```python
from build123d import *

# Parameters (mm, degrees)
SKETCH_1_W               = 8
SKETCH_1_H               = 10
SKETCH_1_R               = 1.5
EXTRUDE_1_DEPTH          = 0.5
SM_START                 = -5
SM_EDGE_FLANGE_1_DEPTH   = 10
SM_EDGE_FLANGE_1_2_DEPTH = 10
SM_EDGE_FLANGE_2_DEPTH   = 10
SM_EDGE_FLANGE_2_2_DEPTH = 10
FILLET_1_R               = 2
SKETCH_18_R              = 1.5
CUT_EXTRUDE_1_DEPTH      = 10


# Read off the part's stored shape, not the designer's step: Ребро-кромка1, Ребро-кромка2
with BuildPart() as part:
    # Sketch 1 → Бобышка-Вытянуть1 (new body)
    with BuildSketch(Plane(origin=(0, 0, 0), x_dir=(1, 0, 0), z_dir=(0, 1, 0))):
        Rectangle(SKETCH_1_W, SKETCH_1_H)
        with Locations(Location((0, 0, 0), (0, 0, 270))):
            Circle(SKETCH_1_R, mode=Mode.SUBTRACT)
    extrude(amount=EXTRUDE_1_DEPTH)

    # Ребро-кромка1 outline → Ребро-кромка1 (cut)
    with BuildSketch(Plane.XY.offset(SM_START)):
        with BuildLine():
            ThreePointArc((-2.75383711, 0), (-3.25383711, 0.133974596), (-3.619862514, 0.5))
            Line((-3.619862514, 0.5), (-4, 0.5))
            Line((-4, 0.5), (-4, 0))
            Line((-4, 0), (-2.75383711, 0))
        make_face()
        with BuildLine():
            ThreePointArc((3.619862514, 0.5), (3.25383711, 0.133974596), (2.75383711, 0))
            Line((2.75383711, 0), (4, 0))
            Line((4, 0), (4, 0.5))
            Line((4, 0.5), (3.619862514, 0.5))
        make_face()
    extrude(amount=SM_EDGE_FLANGE_1_DEPTH, mode=Mode.SUBTRACT)

    # Sm Edge Flange 1 2 outline → Sm Edge Flange 1 2 (add)
    with BuildSketch(Plane.XY.offset(SM_START)):
        with BuildLine():
            Line((-2.129864257, 5.638155725), (-3.693529731, 1.342020143))
            ThreePointArc((-3.693529731, 1.342020143), (-3.750031808, 0.912844257), (-3.619862514, 0.5))
            Line((-3.619862514, 0.5), (-2.75383711, 0.5))
            ThreePointArc((-2.75383711, 0.5), (-3.163413133, 0.713211782), (-3.223683421, 1.171010072))
            Line((-3.223683421, 1.171010072), (-1.660017947, 5.467145653))
            Line((-1.660017947, 5.467145653), (-2.129864257, 5.638155725))
        make_face()
        with BuildLine():
            ThreePointArc((3.223683421, 1.171010072), (3.163413133, 0.713211782), (2.75383711, 0.5))
            Line((2.75383711, 0.5), (3.619862514, 0.5))
            ThreePointArc((3.619862514, 0.5), (3.750031808, 0.912844257), (3.693529731, 1.342020143))
            Line((3.693529731, 1.342020143), (2.129864257, 5.638155725))
            Line((2.129864257, 5.638155725), (1.660017947, 5.467145653))
            Line((1.660017947, 5.467145653), (3.223683421, 1.171010072))
        make_face()
    extrude(amount=SM_EDGE_FLANGE_1_2_DEPTH)

    # Ребро-кромка2 outline → Ребро-кромка2 (cut)
    with BuildSketch(Plane.XY.offset(SM_START)):
        with BuildLine():
            Line((-2.129864257, 5.638155725), (-2.129864257, 4.352580505))
            ThreePointArc((-2.129864257, 4.352580505), (-2.145056504, 4.178932328), (-2.190171636, 4.010560362))
            Line((-2.190171636, 4.010560362), (-1.660017947, 5.467145653))
            Line((-1.660017947, 5.467145653), (-2.129864257, 5.638155725))
        make_face()
        with BuildLine():
            Line((2.129864257, 4.352580505), (2.129864257, 5.638155725))
            Line((2.129864257, 5.638155725), (1.660017947, 5.467145653))
            Line((1.660017947, 5.467145653), (2.190171636, 4.010560362))
            ThreePointArc((2.190171636, 4.010560362), (2.145056504, 4.178932328), (2.129864257, 4.352580505))
        make_face()
    extrude(amount=SM_EDGE_FLANGE_2_DEPTH, mode=Mode.SUBTRACT)

    # Sm Edge Flange 2 2 outline → Sm Edge Flange 2 2 (add)
    with BuildSketch(Plane.XY.offset(SM_START)):
        with BuildLine():
            Line((-2.660017947, 4.181570434), (-2.129864257, 5.638155725))
            Line((-2.129864257, 5.638155725), (-2.129864257, 14.176253525))
            Line((-2.129864257, 14.176253525), (-2.629864257, 14.176253525))
            Line((-2.629864257, 14.176253525), (-2.629864257, 4.352580505))
            ThreePointArc((-2.629864257, 4.352580505), (-2.637460381, 4.265756417), (-2.660017947, 4.181570434))
        make_face()
        with BuildLine():
            Line((2.629864257, 4.352580505), (2.629864257, 14.176253525))
            Line((2.629864257, 14.176253525), (2.129864257, 14.176253525))
            Line((2.129864257, 14.176253525), (2.129864257, 5.638155725))
            Line((2.129864257, 5.638155725), (2.660017947, 4.181570434))
            ThreePointArc((2.660017947, 4.181570434), (2.637460381, 4.265756417), (2.629864257, 4.352580505))
        make_face()
    extrude(amount=SM_EDGE_FLANGE_2_2_DEPTH)

    # Скругление1
    fillet_1_edges = [part.edges().sort_by_distance(p)[0] for p in [
        (-2.379864257, 14.176253525, 5),
        (-2.379864257, 14.176253525, -5),
        (2.379864257, 14.176253525, -5),
        (2.379864257, 14.176253525, 5),
    ]]
    fillet(fillet_1_edges, radius=FILLET_1_R)

    # Эскиз18 → Вырез-Вытянуть1 (cut)
    with BuildSketch(Plane(origin=(2.629864257, 0, 0), x_dir=(0, 0, -1), z_dir=(1, 0, 0))):
        with Locations(Location((0, 9.176253525, 0), (0, 0, 90))):
            Circle(SKETCH_18_R)
    extrude(amount=-CUT_EXTRUDE_1_DEPTH, mode=Mode.SUBTRACT)


solid = part.part
```
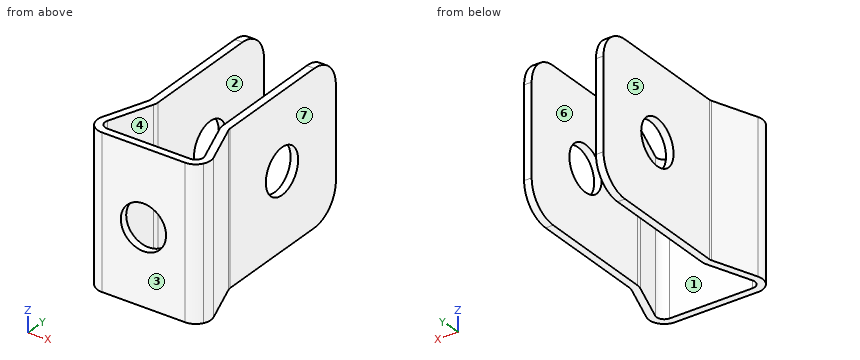
The model under review builds one solid part; all positions refer to its coordinate system, in mm. Face numbers are marked on the shaded views. A direction names the side the tool comes from. Give positions to 0.01 mm unless a question says otherwise; leave off trailing zeros. Order: outer loops, then holes, each group sorted by start corner. A loop starts at its lowest first (then second) coordinate and runs counter-clockwise, first axis right, second up. Notation, with made-up numbers: (83.25, 65) - (104.25, 65) arc R22 ccw to (104.25, 71) - close; hole circle Ø2 at (11, -23). An arc over 180 degrees is marked (long way). Use CSV: the item, a comma, the result in double quotes. Start each with the question number.
Q1. We need section B-B, the plane x = 0. Write out the cut boundary in (y, z).
Q2. To check wall thickness, follow line 1 along X through (y, z) = (8, -3); line 2 along X through (y, z) = (1, -3.5); line 3 along Y through (x, z) = (-2, 2.5). State the ranges of each line that lie inside material, in increasing order. Write a range as [from, to].
Q3. We need section D-D, the plane z = -1. State how many separate pieces and enclosed holes the cut face has, and give its area (3 significant figures).
Q4. We need section A-A, the plane y = 12. Write out the cut boundary in (x, z), and give its area (3 significant figures).
Q5. The part is to be moulded in two halves that separate along Y. For the marked faces 1, 2 and 3, say which applies: +Y half, -Y half, draft (parallel to the pull), parting line (faces both ways), or undercut.
Q6. Clearance check with flat-ended pins moving along their axes: pin 1 Ø5 at (y, z) = (9.18, 0) entering from -X; pin 2 Ø4 at (x, y) = (-2, 6) entering from +Z; pin 3 Ø3 at (y, z) = (11, -0.5) entering from +X. State where each tip first meets the part, or that it passes through.
Q7. Tool access review of the marked faces 4, 5, 6 and 7: name each direction out of +Z, -Z, +X, -X, +Y, -Y from which nothing blocks a thin tool from reaching the whole face with its end or side.
Q8. We need section C-C, the plane z = 2.5. Write out the cut boundary in (x, y), and give its area (3 significant figures).
Outcome:
1,outline,"(0, -5) - (0.5, -5) - (0.5, -1.5) - (0, -1.5) - close; (0, 1.5) - (0.5, 1.5) - (0.5, 5) - (0, 5) - close"
2,line 1,"x = [-2.63, -2.13], [2.13, 2.63]"
2,line 2,"x = [-3.75, -3.25], [3.25, 3.75]"
2,line 3,"y = [0, 0.5]"
3,separate pieces,"4"
3,enclosed holes,"0"
3,area,"13.9 mm^2"
4,outline,"(-2.63, -5) - (-2.13, -5) - (-2.13, 5) - (-2.63, 5) - close; (2.13, -5) - (2.63, -5) - (2.63, 5) - (2.13, 5) - close"
4,area,"10.0 mm^2"
5,face 1,"undercut"
5,face 2,"draft"
5,face 3,"-Y half"
6,pin 1,"stops at x = -2.63"
6,pin 2,"stops at z = 5"
6,pin 3,"stops at x = 2.63"
7,face 4,"+Z, -Z"
7,face 5,"+Z, -Z, -X, +Y"
7,face 6,"+Z, -Z, +Y"
7,face 7,"+Z, -Z, +X, +Y"
8,outline,"(-3.69, 1.34) arc R1 ccw to (-2.75, 0) - (2.75, 0) arc R1 ccw to (3.69, 1.34) - (2.66, 4.18) arc R0.5 cw to (2.63, 4.35) - (2.63, 14.18) - (2.13, 14.18) - (2.13, 4.35) arc R1 ccw to (2.19, 4.01) - (3.22, 1.17) arc R0.5 cw to (2.75, 0.5) - (-2.75, 0.5) arc R0.5 cw to (-3.22, 1.17) - (-2.19, 4.01) arc R1 ccw to (-2.13, 4.35) - (-2.13, 14.18) - (-2.63, 14.18) - (-2.63, 4.35) arc R0.5 cw to (-2.66, 4.18) - close"
8,area,"17.3 mm^2"
